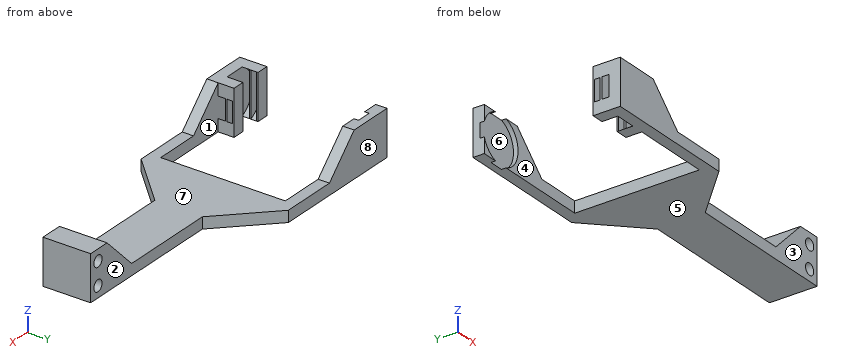
```python
from build123d import *

# Parameters (mm, degrees)
EXTRUSION1_DEPTH        = 20
ESQUISSE3_R             = 2.5
ENL_V_MAT_EXTRU_1_DEPTH = 44
ENL_V_MAT_EXTRU_2_DEPTH = 66
ESQUISSE5_R             = 10.5
ENL_V_MAT_EXTRU_3_DEPTH = 2
EXTRUSION2_DEPTH        = 7
ESQUISSE7_W             = 20
ESQUISSE7_H             = 0.7
EXTRUSION3_DEPTH        = 20
ESQUISSE8_W             = 9.16515139
ESQUISSE8_H             = 7
ENL_V_MAT_EXTRU_4_DEPTH = 21


with BuildPart() as part:
    # Esquisse2 → Extrusion1 (new body)
    with BuildSketch(Plane.XY):
        Polygon((0, 32.5), (0, 27.5), (55, 27.5), (55, -27.5), (0, -27.5), (0, -32.5), (60, -32.5), (82, -10.5), (150, -10.5), (150, 10.5), (82, 10.5), (60, 32.5), align=None)
    extrude(amount=EXTRUSION1_DEPTH)

    # Esquisse3 → Enlèv. mat.-Extru.1 (cut, through all)
    with BuildSketch(Plane.XZ.offset(10.5)):
        with Locations((145.5, 15)):
            Circle(ESQUISSE3_R)
        with Locations((145.5, 5)):
            Circle(ESQUISSE3_R)
    extrude(amount=-ENL_V_MAT_EXTRU_1_DEPTH, mode=Mode.SUBTRACT)

    # Esquisse4 → Enlèv. mat.-Extru.2 (cut, through all)
    with BuildSketch(Plane.XZ.offset(32.5)):
        Polygon((20, 20), (35, 5), (125, 5), (140, 20), align=None)
    extrude(amount=-ENL_V_MAT_EXTRU_2_DEPTH, mode=Mode.SUBTRACT)

    # Esquisse5 → Enlèv. mat.-Extru.3 (cut)
    with BuildSketch(Plane.XZ.offset(-27.5)):
        with Locations((10, 10)):
            Circle(ESQUISSE5_R)
    extrude(amount=-ENL_V_MAT_EXTRU_3_DEPTH, mode=Mode.SUBTRACT)

    # Esquisse6 → Extrusion2 (add)
    with BuildSketch(Plane(origin=(0, -27.5, 0), x_dir=(1, 0, 0), z_dir=(0, 1, 0))):
        with BuildLine():
            Line((14.582575695, 0), (20, 0))
            Line((20, 0), (20, -5.417424305))
            ThreePointArc((20, -5.417424305), (17.778174593, -2.221825407), (14.582575695, 0))
        make_face()
        with BuildLine():
            Line((0, 0), (5.417424305, 0))
            ThreePointArc((5.417424305, 0), (2.221825407, -2.221825407), (0, -5.417424305))
            Line((0, -5.417424305), (0, 0))
        make_face()
        with BuildLine():
            Line((0, -20), (5.417424305, -20))
            ThreePointArc((5.417424305, -20), (2.221825407, -17.778174593), (0, -14.582575695))
            Line((0, -14.582575695), (0, -20))
        make_face()
        with BuildLine():
            Line((20, -14.582575695), (20, -20))
            Line((20, -20), (14.582575695, -20))
            ThreePointArc((14.582575695, -20), (17.778174593, -17.778174593), (20, -14.582575695))
        make_face()
    extrude(amount=EXTRUSION2_DEPTH)

    # Esquisse7 → Extrusion3 (add)
    with BuildSketch(Plane.ZY):
        with Locations((10, -20.85)):
            Rectangle(ESQUISSE7_W, ESQUISSE7_H)
        with Locations((10, -24)):
            Rectangle(ESQUISSE7_W, ESQUISSE7_H)
    extrude(amount=-EXTRUSION3_DEPTH)

    # Esquisse8 → Enlèv. mat.-Extru.4 (cut, through all)
    with BuildSketch(Plane.XY.offset(20)):
        with Locations((10, -24)):
            Rectangle(ESQUISSE8_W, ESQUISSE8_H)
    extrude(amount=-ENL_V_MAT_EXTRU_4_DEPTH, mode=Mode.SUBTRACT)


solid = part.part
```
Model file for the job. Use its own axes, mm. Face numbers are marked on the shaded views. A direction names the side the tool comes from. Coordinates: 2 decimals unless noted, no trailing zeros. Write each loop counter-clockwise with the first axis right and the second up, starting at its lowest first coordinate (ties: lowest second). Pieces come first, ordered by that corner, then holes. Notation, with made-up numbers: (-1, 3) - (9, 3) arc R16 ccw to (9, 22) - close; hole circle Ø11 at (13, 17.25). An arc over 180 degrees is marked (long way). Use a Markdown table: item, result. Add a question column.
Item 1: Two-plate mould, pull along Z, no slides. Class the marked faces 6, 7 and 8: pulls with the +Z half, pulls with the -Z half, needs draft (parallel to the pull), parting line crosses it, or undercut.
Item 2: Drop flat-ended pins along their axis: pin 1 (1 mm diameter, centred on y = 6, z = 15, fed in from -X); pin 2 (10 mm diameter, centred on x = 95, z = 5, fed in from -Y); pin 3 (12 mm diameter, centred on x = 74, z = 2, fed in from +Y). Give the stop position or say it passes through.
Item 3: Band-saw the part on C-C, the plane z = 10.5. Give the number of separate pieces and of enclosed holes in the cut face, and give its area (3 significant figures).
Item 4: 3-axis set-ups, long thin cutter, end or side, ignore diameter. For the marked faces 1, 2, 3, 4 and 5: which of +Z, -Z, +X, -X, +Y, -Y reach the whole face in a straight line?
Item 5: Band-saw the part on B-B, the plane y = 6. Write the cut outline in (x, z), and give its area (3 significant figures).
Item 6: Band-saw the part on A-A, the plane x = 145.5. Write the cut outline in (y, z), and give its area (3 significant figures).
Item 7: Band-saw the part on D-D, the plane y = -15. Write the cut outline in (x, z).
Item 8: Drill centre lines: line 1 along Z through (x, y) = (145.5, -3.5); line 2 along Y through (x, z) = (28, 2.5); line 3 along Y through (x, z) = (9, 15.5). Where is each one in solid material? Low to high.
A:
| question | item | result |
|---|---|---|
| 1 | face 6 | undercut |
| 1 | face 7 | pulls with the +Z half |
| 1 | face 8 | needs draft |
| 2 | pin 1 | stops at x = 134.5 |
| 2 | pin 2 | stops at y = -10.5 |
| 2 | pin 3 | stops at y = 24.5 |
| 3 | separate pieces | 7 |
| 3 | enclosed holes | 0 |
| 3 | area | 679 mm² |
| 4 | face 1 | none |
| 4 | face 2 | +Z, -Z, +X, +Y |
| 4 | face 3 | +Z, -Z, +X, -Y |
| 4 | face 4 | +Z, -Z, -X |
| 4 | face 5 | -Z, +X, -X, +Y, -Y |
| 5 | outline | (55, 0) - (150, 0) - (150, 20) - (140, 20) - (125, 5) - (55, 5) - close; hole circle Ø5 at (145.5, 5); hole circle Ø5 at (145.5, 15) |
| 5 | area | 698 mm² |
| 6 | outline | (-10.5, 0) - (10.5, 0) - (10.5, 2.5) - (-10.5, 2.5) - close; (-10.5, 7.5) - (10.5, 7.5) - (10.5, 12.5) - (-10.5, 12.5) - close; (-10.5, 17.5) - (10.5, 17.5) - (10.5, 20) - (-10.5, 20) - close |
| 6 | area | 210 mm² |
| 7 | outline | (55, 0) - (77.5, 0) - (77.5, 5) - (55, 5) - close |
| 8 | line 1 | z = 0 to 2.5, 7.5 to 12.5, 17.5 to 20 |
| 8 | line 2 | y = -32.5 to -27.5, 27.5 to 32.5 |
| 8 | line 3 | y = -32.5 to -27.5, 29.5 to 32.5 |
